Drawing for the job (mm, zero at the part's lowest x, y, z). A direction names the side the tool comes from. Round coordinates to 2 decimals unless told otherwise and drop trailing zeros. Loops run counter-clockwise (first coordinate to the right, second up) from the corner with the lowest first, then second, coordinate; pieces in that order, holes last. Notation, with made-up numbers: (35, -18.75) - (88, -18.75) arc R25 cw to (88, 12.25) - close; hole circle Ø11 at (31.5, -4). An arc over 180 degrees is marked (long way). Put each result on its own line as item: value.
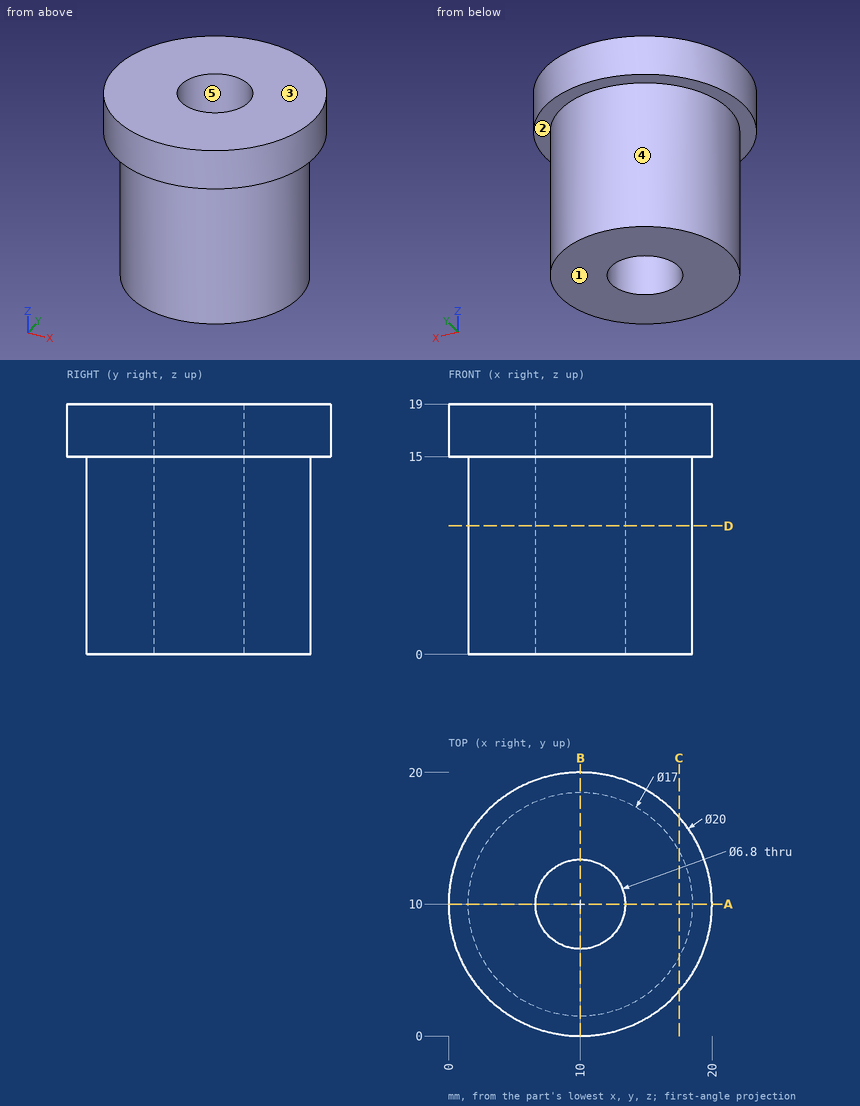
1. Two-plate mould, pull along X, no slides. Class the marked faces 3, 4 and 5: pulls with the +X half, pulls with the -X half, needs draft (parallel to the pull), parting line crosses it, or undercut.
A:
face 3: needs draft
face 4: parting line crosses it
face 5: undercut
2. Band-saw the part on D-D (z = 9.75). List the corners of the cut face in (x, y), plus the area to 3 significant figures.
A:
outline: circle Ø17 at (10, 10); hole circle Ø6.8 at (10, 10)
area: 191 mm²
3. Probe line 1 along Y through (x, z) = (10, 15.25); line 2 along Y through (x, z) = (10, 4); line 3 along Z through (x, y) = (3.75, 17). List the from-to ranges inside material, lowest first. Write a range as [from, to].
A:
line 1: y = [0, 6.6], [13.4, 20]
line 2: y = [1.5, 6.6], [13.4, 18.5]
line 3: z = [15, 19]
4. Tool access for the marked faces 1 and 2: list every direction of +Z, -Z, +X, -X, +Y, -Y with a clear straight run to the whole face (end or side of a thin tool).
A:
face 1: -Z, +X, -X, +Y, -Y
face 2: -Z
5. Band-saw the part on A-A (y = 10). List the corners of the cut face in (x, z), plus the area to 3 significant figures.
A:
outline: (0, 15) - (1.5, 15) - (1.5, 0) - (6.6, 0) - (6.6, 19) - (0, 19) - close; (13.4, 0) - (18.5, 0) - (18.5, 15) - (20, 15) - (20, 19) - (13.4, 19) - close
area: 206 mm²
6. Pin check, flat tips, straight feed: P1, Ø10, axis at y = 12, z = 5.5, coming from the -X side; P2, Ø1.5, axis at x = 5, z = 17, coming from the -Y side; P3, Ø1, axis at x = 6, z = 5.5, coming from the +Y side. Stop position of each tip, or through.
A:
P1: stops at x = 1.5
P2: stops at y = 0.95
P3: stops at y = 17.75
7. Band-saw the part on C-C (x = 17.5). List the corners of the cut face in (y, z).
A:
outline: (3.39, 15) - (6, 15) - (6, 0) - (14, 0) - (14, 15) - (16.61, 15) - (16.61, 19) - (3.39, 19) - close
